from build123d import *

# Parameters (mm, degrees)
CROQUIS1_R              = 1.6
SALIENTE_EXTRUIR1_DEPTH = 2
CROQUIS2_W              = 29.5
CROQUIS2_H              = 13
SALIENTE_EXTRUIR2_DEPTH = 7.2
CROQUIS3_W              = 10.1
CROQUIS3_H              = 8
SALIENTE_EXTRUIR3_DEPTH = 9.9
SALIENTE_EXTRUIR4_DEPTH = 4.5
CROQUIS5_W              = 10.1
CROQUIS5_H              = 1.2
SALIENTE_EXTRUIR5_DEPTH = 6
CROQUIS6_W              = 8
CROQUIS6_H              = 4.8
SALIENTE_EXTRUIR6_DEPTH = 5.9


with BuildPart() as part:
    # Croquis1 → Saliente-Extruir1 (new body)
    with BuildSketch(Plane.XY):
        with BuildLine():
            Line((18.5, -3.75), (-18.5, -3.75))
            ThreePointArc((-18.5, -3.75), (-22.25, 0), (-18.5, 3.75))
            Line((-18.5, 3.75), (18.5, 3.75))
            ThreePointArc((18.5, 3.75), (22.25, 0), (18.5, -3.75))
        make_face()
        with Locations((-18.5, 0)):
            Circle(CROQUIS1_R, mode=Mode.SUBTRACT)
        with Locations((18.5, 0)):
            Circle(CROQUIS1_R, mode=Mode.SUBTRACT)
    extrude(amount=SALIENTE_EXTRUIR1_DEPTH)

    # Croquis2 → Saliente-Extruir2 (add)
    with BuildSketch(Plane.XY):
        Rectangle(CROQUIS2_W, CROQUIS2_H)
    extrude(amount=SALIENTE_EXTRUIR2_DEPTH)

    # Croquis3 → Saliente-Extruir3 (add)
    with BuildSketch(Plane.XY.offset(7.2)):
        with BuildLine():
            ThreePointArc((-5.8, 4.2), (-6.312563133, 5.437436867), (-7.55, 5.95))
            Line((-7.55, 5.95), (-13, 5.95))
            ThreePointArc((-13, 5.95), (-14.237436867, 5.437436867), (-14.75, 4.2))
            Line((-14.75, 4.2), (-14.75, -4.2))
            ThreePointArc((-14.75, -4.2), (-14.237436867, -5.437436867), (-13, -5.95))
            Line((-13, -5.95), (-7.55, -5.95))
            ThreePointArc((-7.55, -5.95), (-6.312563133, -5.437436867), (-5.8, -4.2))
            Line((-5.8, -4.2), (-5.8, -4))
            Line((-5.8, -4), (-5.8, 4))
            Line((-5.8, 4), (-5.8, 4.2))
        make_face()
        with Locations((-0.75, 0)):
            Rectangle(CROQUIS3_W, CROQUIS3_H)
        with BuildLine():
            Line((4.3, 4.2), (4.3, 4))
            Line((4.3, 4), (4.3, -4))
            Line((4.3, -4), (4.3, -4.2))
            ThreePointArc((4.3, -4.2), (4.812563133, -5.437436867), (6.05, -5.95))
            Line((6.05, -5.95), (13, -5.95))
            ThreePointArc((13, -5.95), (14.237436867, -5.437436867), (14.75, -4.2))
            Line((14.75, -4.2), (14.75, 4.2))
            ThreePointArc((14.75, 4.2), (14.237436867, 5.437436867), (13, 5.95))
            Line((13, 5.95), (6.05, 5.95))
            ThreePointArc((6.05, 5.95), (4.812563133, 5.437436867), (4.3, 4.2))
        make_face()
    extrude(amount=SALIENTE_EXTRUIR3_DEPTH)

    # Croquis4 → Saliente-Extruir4 (add)
    with BuildSketch(Plane.XY.offset(17.1)):
        with BuildLine():
            Line((-5.8, -4), (-5.8, 4))
            Line((-5.8, 4), (-5.8, 4.2))
            ThreePointArc((-5.8, 4.2), (-6.312563133, 5.437436867), (-7.55, 5.95))
            Line((-7.55, 5.95), (-13, 5.95))
            ThreePointArc((-13, 5.95), (-14.237436867, 5.437436867), (-14.75, 4.2))
            Line((-14.75, 4.2), (-14.75, -4.2))
            ThreePointArc((-14.75, -4.2), (-14.237436867, -5.437436867), (-13, -5.95))
            Line((-13, -5.95), (-7.55, -5.95))
            ThreePointArc((-7.55, -5.95), (-6.312563133, -5.437436867), (-5.8, -4.2))
            Line((-5.8, -4.2), (-5.8, -4))
        make_face()
        with BuildLine():
            Line((4.3, 4), (4.3, -4))
            Line((4.3, -4), (4.3, -4.2))
            ThreePointArc((4.3, -4.2), (4.812563133, -5.437436867), (6.05, -5.95))
            Line((6.05, -5.95), (13, -5.95))
            ThreePointArc((13, -5.95), (14.237436867, -5.437436867), (14.75, -4.2))
            Line((14.75, -4.2), (14.75, 4.2))
            ThreePointArc((14.75, 4.2), (14.237436867, 5.437436867), (13, 5.95))
            Line((13, 5.95), (6.05, 5.95))
            ThreePointArc((6.05, 5.95), (4.812563133, 5.437436867), (4.3, 4.2))
            Line((4.3, 4.2), (4.3, 4))
        make_face()
    extrude(amount=SALIENTE_EXTRUIR4_DEPTH)

    # Croquis5 → Saliente-Extruir5 (add)
    with BuildSketch(Plane.XZ.offset(6.5)):
        with Locations((0, 3.9)):
            Rectangle(CROQUIS5_W, CROQUIS5_H)
    extrude(amount=SALIENTE_EXTRUIR5_DEPTH)

    # Croquis6 → Saliente-Extruir6 (add)
    with BuildSketch(Plane.XZ.offset(6.5)):
        with Locations((0, 6.9)):
            Rectangle(CROQUIS6_W, CROQUIS6_H)
    extrude(amount=SALIENTE_EXTRUIR6_DEPTH)


solid = part.part
The listing builds one solid part. Answer for the finished solid, in the listing's coordinates (mm). A direction names the side the tool comes from. Coordinates: 2 decimals unless noted, no trailing zeros. Loops run counter-clockwise (first coordinate to the right, second up) from the corner with the lowest first, then second, coordinate; pieces in that order, holes last. Notation, with made-up numbers: M 16,1.25 L 20,1.25 A22 cw 20,29.25 Z; hole C 5,1 d2. An arc over 180 degrees is marked long. Answer in a Markdown table with one row per item.
1) Find section A-A (z = 18.25). Determine the outline of the cut face in (x, y), then the cut area to 3 significant figures.
Answers below:
| item | result |
|---|---|
| outline | M -14.75,-4.2 A1.75 ccw -13,-5.95 L -7.55,-5.95 A1.75 ccw -5.8,-4.2 L -5.8,4.2 A1.75 ccw -7.55,5.95 L -13,5.95 A1.75 ccw -14.75,4.2 Z; M 4.3,-4.2 A1.75 ccw 6.05,-5.95 L 13,-5.95 A1.75 ccw 14.75,-4.2 L 14.75,4.2 A1.75 ccw 13,5.95 L 6.05,5.95 A1.75 ccw 4.3,4.2 Z |
| area | 226 mm^2 |
2) Determine the mould class of faces 4 (the flat face through (-5.05, -9, 4)), 5 (the flat face through (4.3, 0, 19)), 6 (the cylindrical face through (14.224, -5.451, 14.299)) for opening direction X: released by +X, released by -X, zero draft, split by the parting line, or undercut.
Answers below:
| item | result |
|---|---|
| face 4 | released by -X |
| face 5 | undercut |
| face 6 | released by +X |
3) Find section C-C (x = 2.5). Determine the outline of the cut face in (y, z), then the cut area to 3 significant figures.
Answers below:
| item | result |
|---|---|
| outline | M -12.5,3.3 L -6.5,3.3 L -6.5,0 L 6.5,0 L 6.5,7.2 L 4,7.2 L 4,17.1 L -4,17.1 L -4,7.2 L -6.5,7.2 L -6.5,9.3 L -12.4,9.3 L -12.4,4.5 L -12.5,4.5 Z |
| area | 208 mm^2 |
4) Given pin 1 (1 mm diameter, centred on x = 16.5, z = 1, fed in from -Y); pin 2 (2 mm diameter, centred on x = -17, z = 1, fed in from +Y); pin 3 (4 mm diameter, centred on y = -10, z = 8, fed in from -X); pin 4 (1.5 mm diameter, centred on x = 5.5, y = 4.5, fed in from -Z), each flat-ended and moving along its own axis, determine where each tip first touches the part or whether it passes through.
Answers below:
| item | result |
|---|---|
| pin 1 | y = -3.75 |
| pin 2 | y = 3.75 |
| pin 3 | x = -4 |
| pin 4 | z = 0 |
5) Find the intervals of material crossed by probe 1 along X at (y, z) = (-0.5, 1.5); probe 2 along Y at (x, z) = (-18.5, 1.1); probe 3 along X at (y, z) = (-2.5, 18.5), in increasing order.
Answers below:
| item | result |
|---|---|
| probe 1 | -22.22 to -20.02, -16.98 to 16.98, 20.02 to 22.22 |
| probe 2 | -3.75 to -1.6, 1.6 to 3.75 |
| probe 3 | -14.75 to -5.8, 4.3 to 14.75 |
6) Find section B-B (y = 0). Determine the outline of the cut face in (x, z).
Answers below:
| item | result |
|---|---|
| outline | M -22.25,0 L -20.1,0 L -20.1,2 L -22.25,2 Z; M -16.9,0 L 16.9,0 L 16.9,2 L 14.75,2 L 14.75,21.6 L 4.3,21.6 L 4.3,17.1 L -5.8,17.1 L -5.8,21.6 L -14.75,21.6 L -14.75,2 L -16.9,2 Z; M 20.1,0 L 22.25,0 L 22.25,2 L 20.1,2 Z |
7) Which of the six approach directions +Z, -Z, +X, -X, +Y, -Y give full straight-line access (tool end or side, diameter ignored) to faces 1 (the flat face through (-17, -3.75, 1)), 2 (the flat face through (-17, -1, 2)), 3 (the flat face through (4, -9, 7))?
Answers below:
| item | result |
|---|---|
| face 1 | +Z, -Z, -X, -Y |
| face 2 | +Z, -X, +Y, -Y |
| face 3 | +Z, +X, -Y |
8) Find section D-D (z = 10.75). Determine the outline of the cut face in (x, y), then the cut area to 3 significant figures.
Answers below:
| item | result |
|---|---|
| outline | M -14.75,-4.2 A1.75 ccw -13,-5.95 L -7.55,-5.95 A1.75 ccw -5.8,-4.2 L -5.8,-4 L 4.3,-4 L 4.3,-4.2 A1.75 ccw 6.05,-5.95 L 13,-5.95 A1.75 ccw 14.75,-4.2 L 14.75,4.2 A1.75 ccw 13,5.95 L 6.05,5.95 A1.75 ccw 4.3,4.2 L 4.3,4 L -5.8,4 L -5.8,4.2 A1.75 ccw -7.55,5.95 L -13,5.95 A1.75 ccw -14.75,4.2 Z |
| area | 306 mm^2 |
